from build123d import *

# Parameters (mm, degrees)
SKETCH1_W                      = 127
SKETCH1_H                      = 63.5
BOSS_EXTRUDE1_DEPTH            = 6.35
F_9_0_196_DIAMETER_HOLE1_D     = 4.9784
F_9_0_196_DIAMETER_HOLE1_DEPTH = 70.104
F_9_0_196_DIAMETER_HOLE1_TIP   = 1.495662253
F_9_0_196_DIAMETER_HOLE2_D     = 4.9784
F_9_0_196_DIAMETER_HOLE2_DEPTH = 70.104
F_9_0_196_DIAMETER_HOLE2_TIP   = 1.495662253
Z_0_413_DIAMETER_HOLE1_D       = 10.4902
Z_0_413_DIAMETER_HOLE1_DEPTH   = 70.104
Z_0_413_DIAMETER_HOLE1_TIP     = 3.151574033


with BuildPart() as part:
    # Sketch1 → Boss-Extrude1 (new body)
    with BuildSketch(Plane(origin=(0, 0, 0), x_dir=(0, 0, -1), z_dir=(1, 0, 0))):
        Rectangle(SKETCH1_W, SKETCH1_H)
    extrude(amount=BOSS_EXTRUDE1_DEPTH)

    # #9 (0.196) Diameter Hole1
    with Locations(Plane.ZY):
        with Locations((57.15, -22.225), (6.35, -22.225)):
            Hole(F_9_0_196_DIAMETER_HOLE1_D / 2, depth=F_9_0_196_DIAMETER_HOLE1_DEPTH)
            with Locations((0, 0, -(F_9_0_196_DIAMETER_HOLE1_DEPTH + F_9_0_196_DIAMETER_HOLE1_TIP / 2))):  # 118° drill point
                Cone(0, F_9_0_196_DIAMETER_HOLE1_D / 2, F_9_0_196_DIAMETER_HOLE1_TIP, mode=Mode.SUBTRACT)

    # #9 (0.196) Diameter Hole2
    with Locations(Plane.ZY):
        with Locations((-57.15, -25.4), (-19.05, -25.4), (-19.05, 25.4), (-57.15, 25.4)):
            Hole(F_9_0_196_DIAMETER_HOLE2_D / 2, depth=F_9_0_196_DIAMETER_HOLE2_DEPTH)
            with Locations((0, 0, -(F_9_0_196_DIAMETER_HOLE2_DEPTH + F_9_0_196_DIAMETER_HOLE2_TIP / 2))):  # 118° drill point
                Cone(0, F_9_0_196_DIAMETER_HOLE2_D / 2, F_9_0_196_DIAMETER_HOLE2_TIP, mode=Mode.SUBTRACT)

    # Z (0.413) Diameter Hole1
    with Locations(Plane.ZY):
        with Locations((31.75, -12.7)):
            Hole(Z_0_413_DIAMETER_HOLE1_D / 2, depth=Z_0_413_DIAMETER_HOLE1_DEPTH)
            with Locations((0, 0, -(Z_0_413_DIAMETER_HOLE1_DEPTH + Z_0_413_DIAMETER_HOLE1_TIP / 2))):  # 118° drill point
                Cone(0, Z_0_413_DIAMETER_HOLE1_D / 2, Z_0_413_DIAMETER_HOLE1_TIP, mode=Mode.SUBTRACT)


solid = part.part
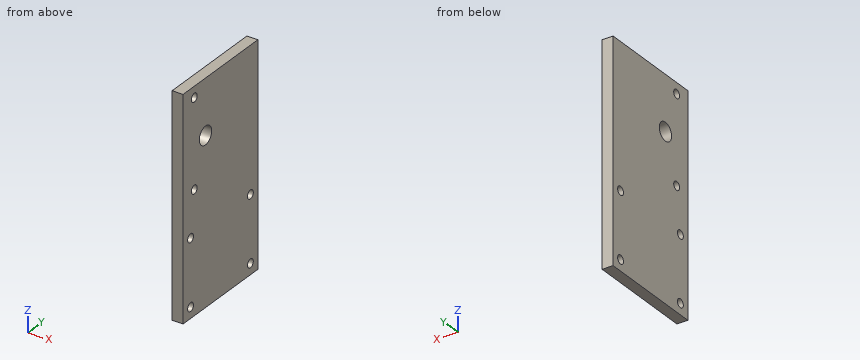
Model file for the job. Use its own axes, mm. Round coordinates to 2 decimals unless told otherwise and drop trailing zeros. Loops run counter-clockwise (first coordinate to the right, second up) from the corner with the lowest first, then second, coordinate; pieces in that order, holes last. Notation, with made-up numbers: (26, 23) -> (52, 23) arc R31 ccw to (52, 56) -> close; hole circle Ø8 at (78, 49.25). An arc over 180 degrees is marked (long way). Answer as CSV lines item,"result". Start each with the question number.
1) Pin check, flat tip, straight feed: P1, Ø3, axis at y = -25.4, z = -57.15, coming from the +X side. Stop position of the tip, or through.
2) Slice it at C-C (y = -12.7). List the corners of the cut face in (x, z).
3) Slice it at B-B (z = 31.75). List the corners of the cut face in (x, y).
4) Slice it at A-A (y = 25.4). List the corners of the cut face in (x, z), plus the area to 3 significant figures.
5) Slice it at D-D (z = -57.15). List the corners of the cut face in (x, y), plus the area to 3 significant figures.
6) Probe line 1 along Y through (x, z) = (5, -19.05); line 2 along Z through (x, y) = (4.5, -25); line 3 along Z through (x, y) = (2, -20.5). List the from-to ranges inside material, lowest first.
Filled in:
1,P1,"passes through"
2,outline,"(0, -63.5) -> (6.35, -63.5) -> (6.35, 26.5) -> (0, 26.5) -> close; (0, 37) -> (6.35, 37) -> (6.35, 63.5) -> (0, 63.5) -> close"
3,outline,"(0, -31.75) -> (6.35, -31.75) -> (6.35, -17.95) -> (0, -17.95) -> close; (0, -7.45) -> (6.35, -7.45) -> (6.35, 31.75) -> (0, 31.75) -> close"
4,outline,"(0, -63.5) -> (6.35, -63.5) -> (6.35, -59.64) -> (0, -59.64) -> close; (0, -54.66) -> (6.35, -54.66) -> (6.35, -21.54) -> (0, -21.54) -> close; (0, -16.56) -> (6.35, -16.56) -> (6.35, 63.5) -> (0, 63.5) -> close"
4,area,"743 mm2"
5,outline,"(0, -31.75) -> (6.35, -31.75) -> (6.35, -27.89) -> (0, -27.89) -> close; (0, -22.91) -> (6.35, -22.91) -> (6.35, 22.91) -> (0, 22.91) -> close; (0, 27.89) -> (6.35, 27.89) -> (6.35, 31.75) -> (0, 31.75) -> close"
5,area,"340 mm2"
6,line 1,"y = -31.75 to -27.89, -22.91 to 22.91, 27.89 to 31.75"
6,line 2,"z = -63.5 to -59.61, -54.69 to -21.51, -16.59 to 63.5"
6,line 3,"z = -63.5 to 4.56, 8.14 to 55.36, 58.94 to 63.5"
